Print and shaded views of the part. All mm, measured from the part's lowest x, y and z. A direction names the side the tool comes from. Give positions to 0.01 mm unless a question says otherwise; leave off trailing zeros. Write each loop counter-clockwise with the first axis right and the second up, starting at its lowest first coordinate (ties: lowest second). Pieces come first, ordered by that corner, then holes.
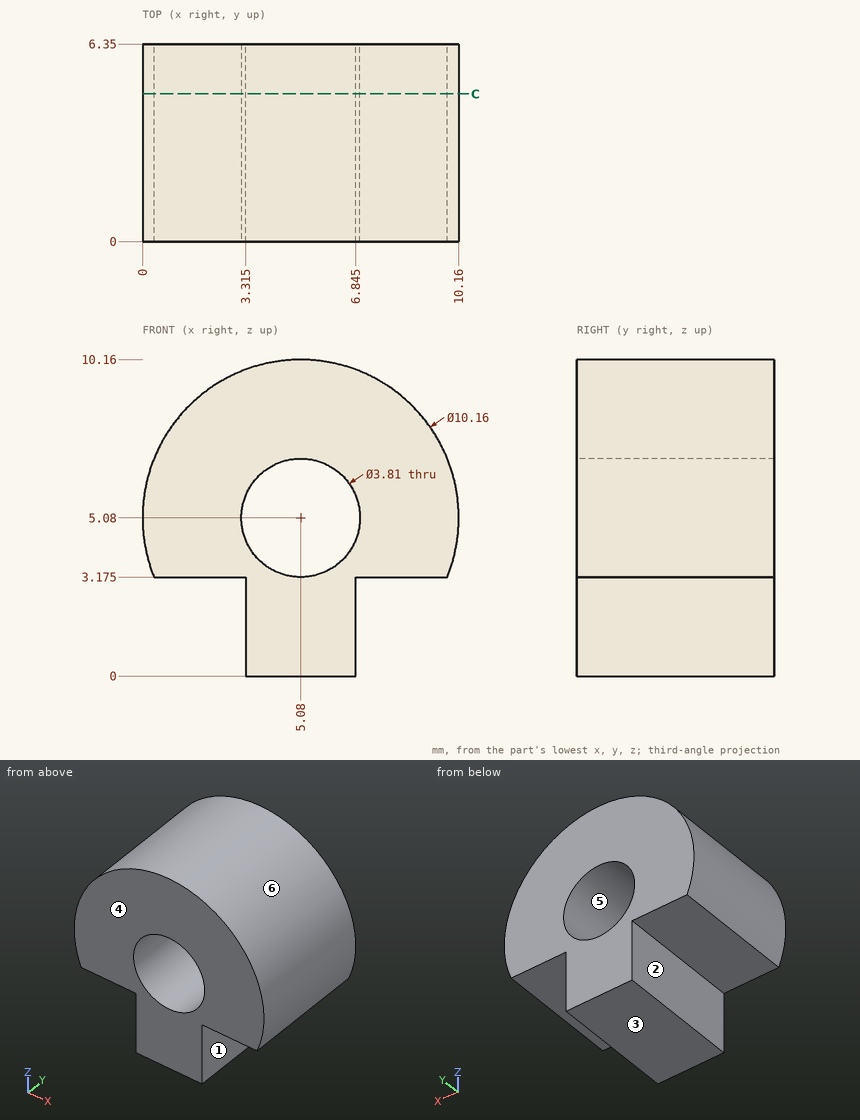
1. Mould opens along X. For the marked faces 4, 5 and 6 say: pulls with the +X half, pulls with the -X half, needs draft (parallel to the pull), parting line crosses it, or undercut.
2. Drill centre lines: line 1 along X through (y, z) = (3, 5.08) (1 decimal); line 2 along X through (y, z) = (4.5, 1.5) (1 decimal). Where is each one in solid material? Low to high.
3. Saw through at C-C on y = 4.75. Give the cut face in (x, z) (1 decimal).
4. Drop flat-ended pins along their axis: pin 1 (1 mm diameter, centred on x = 4, z = 5.5, fed in from +Y); pin 2 (2.5 mm diameter, centred on y = 3.5, z = 1, fed in from -X) (1 decimal); pin 3 (2.5 mm diameter, centred on y = 3, z = 1, fed in from +X) (1 decimal); pin 4 (3 mm diameter, centred on y = 5.5, z = 2, fed in from +X). Give the stop position or say it passes through.
5. 3-axis set-ups, long thin cutter, end or side, ignore diameter. For the marked faces 1, 2 and 3: which of +Z, -Z, +X, -X, +Y, -Y reach the whole face in a straight line?
Outcome:
1. face 4: needs draft
1. face 5: undercut
1. face 6: parting line crosses it
2. line 1: x = 0 to 3.2, 7 to 10.2
2. line 2: x = 3.3 to 6.8
3. outline: (0.4, 3.2) - (3.3, 3.2) - (3.3, 0) - (6.8, 0) - (6.8, 3.2) - (9.8, 3.2) arc R5.1 ccw (long way) to start; hole circle Ø3.8 at (5.1, 5.1)
4. pin 1: passes through
4. pin 2: stops at x = 3.3
4. pin 3: stops at x = 6.8
4. pin 4: stops at x = 9.91
5. face 1: -Z, +X, +Y, -Y
5. face 2: -Z, -X, +Y, -Y
5. face 3: -Z, +X, -X, +Y, -Y
